Can you work these out from the model? Positions are in its coordinate system, mm. A direction names the side the tool comes from. Round coordinates to 2 decimals unless told otherwise and drop trailing zeros. Order: outer loops, then holes, each group sorted by start corner. A loop starts at its lowest first (then second) coordinate and runs counter-clockwise, first axis right, second up. Notation, with made-up numbers: (2.5, -25.75) -> (10.5, -25.75) arc R18 cw to (10.5, -1.75) -> close; hole circle Ø1 at (81.5, 14). An arc over 180 degrees is marked (long way). One line per item, written item: value.
```python
from build123d import *

# Parameters (mm, degrees)
F0_R     = 15.875
F1_DEPTH = 38.1
F2_W     = 9.652
F2_H     = 9.652
F3_DEPTH = 9.652
F4_R     = 9.0043
F5_DEPTH = 17.78
F7_DEPTH = 8.89


with BuildPart() as f1:
    # F0 (on Top) → F1 (new body)
    with BuildSketch(Plane.XY):
        Circle(F0_R)
    extrude(amount=-F1_DEPTH)

    # F2 (on face) → F3 (cut)
    with BuildSketch(Plane(origin=(0, 0, -38.1), x_dir=(1, 0, 0), z_dir=(0, 0, -1))):
        Rectangle(F2_W, F2_H)
    extrude(amount=-F3_DEPTH, mode=Mode.SUBTRACT)

    # F4 (on face) → F5 (cut)
    with BuildSketch(Plane.XY):
        Circle(F4_R)
    extrude(amount=-F5_DEPTH, mode=Mode.SUBTRACT)

    # F6 (on face) → F7 (cut)
    with BuildSketch(Plane.XY.offset(-17.78)):
        with BuildLine():
            Line((5.571118, 7.0739), (-5.571118, 7.0739))
            ThreePointArc((-5.571118, 7.0739), (-9.0043, 0), (-5.571118, -7.0739))
            Line((-5.571118, -7.0739), (5.571118, -7.0739))
            ThreePointArc((5.571118, -7.0739), (8.100662, -3.931501), (9.0043, 0))
            ThreePointArc((9.0043, 0), (8.100662, 3.931501), (5.571118, 7.0739))
        make_face()
    extrude(amount=-F7_DEPTH, mode=Mode.SUBTRACT)


solid = f1.part
```
Q1. On a 3-axis mill with a long thin cutter (end or side, diameter ignored), from which of +Z, -Z, +X, -X, +Y, -Y can I reach the whole of each face in a straight line? I mean faces 5 (the face through (0, -7.074, -22)), 6 (the face through (7, 0, -38.1)), 7 (the face through (0, 0, -28.448)). Say none if no direction works.
Answers below:
face 5: +Z
face 6: -Z, +X, -X, +Y, -Y
face 7: -Z
Q2. I want a section at D-D on z = -35. List the corners of the cut face in (x, y) for me (3 decimals), plus the area to 3 significant figures.
Answers below:
outline: circle Ø31.75 at (0, 0); hole (-4.826, -4.826) -> (4.826, -4.826) -> (4.826, 4.826) -> (-4.826, 4.826) -> close
area: 699 mm^2
Q3. I want a section at A-A on x = 0. List the corners of the cut face in (y, z) for me (3 decimals).
Answers below:
outline: (-15.875, -38.1) -> (-4.826, -38.1) -> (-4.826, -28.448) -> (4.826, -28.448) -> (4.826, -38.1) -> (15.875, -38.1) -> (15.875, 0) -> (9.004, 0) -> (9.004, -17.78) -> (7.074, -17.78) -> (7.074, -26.67) -> (-7.074, -26.67) -> (-7.074, -17.78) -> (-9.004, -17.78) -> (-9.004, 0) -> (-15.875, 0) -> close
Q4. We'd pull the mould along X, two halves only. Please class faces 1 (the face through (0, 8, -17.78)), 2 (the face through (0, 0, -26.67)), 3 (the face through (-3.441, -15.497, -18.783)), 4 (the face through (7, -7, 0)): released by +X, released by -X, zero draft, split by the parting line, or undercut.
Answers below:
face 1: undercut
face 2: undercut
face 3: split by the parting line
face 4: zero draft
Q5. I want a section at B-B on z = -18.5. List the corners of the cut face in (x, y) for me (3 decimals).
Answers below:
outline: circle Ø31.75 at (0, 0); hole (-5.571, -7.074) -> (5.571, -7.074) arc R9.004 ccw to (9.004, 0) arc R9.004 ccw to (5.571, 7.074) -> (-5.571, 7.074) arc R9.004 ccw to start
Q6. Please list where these lines run through material, in increasing order: line 1 along Y through (x, z) = (0, -5) (3 decimals); line 2 along X through (y, z) = (-2, -21.5); line 3 along Z through (x, y) = (2.5, 8.5).
Answers below:
line 1: -15.875 to -9.004, 9.004 to 15.875
line 2: -15.75 to -8.78, 8.78 to 15.75
line 3: -38.1 to -17.78
Q7. I want a section at C-C on y = 4. List the corners of the cut face in (x, z) for me, plus the area to 3 significant figures.
Answers below:
outline: (-15.36, -38.1) -> (-4.83, -38.1) -> (-4.83, -28.45) -> (4.83, -28.45) -> (4.83, -38.1) -> (15.36, -38.1) -> (15.36, 0) -> (8.07, 0) -> (8.07, -26.67) -> (-8.07, -26.67) -> (-8.07, 0) -> (-15.36, 0) -> close
area: 647 mm^2
Q8. Will these pins go through, and if not, where does the flat tip stop? pin 1 Ø1 at (x, y) = (1, 8) entering from +Z; pin 2 Ø5 at (y, z) = (-8.5, -20) entering from -X; pin 3 Ø5 at (y, z) = (-5, -7.5) entering from -X.
Answers below:
pin 1: z = -17.78
pin 2: x = -14.7
pin 3: x = -15.68
